Read the model definition and answer for the solid it produces. Units are mm, in the model's axes. A direction names the side the tool comes from. Give positions to 0.01 mm unless a question says otherwise; leave off trailing zeros. Order: outer loops, then holes, each group sorted by start corner. A loop starts at its lowest first (then second) coordinate and runs counter-clockwise, first axis right, second up. Notation, with made-up numbers: M -9.5,-30.75 L 15.5,-30.75 A27 ccw 15.5,-7.75 Z; hole C -32.5,58 d4. An arc over 180 degrees is marked long. Write item = value, one per line. Start each with the question number.
from build123d import *

# Parameters (mm, degrees)
SKETCH_1_W          = 132
SKETCH_1_H          = 40.05
SKETCH_1_R          = 1.6
EXTRUDE_1_DEPTH     = 3
FILLET_1_R          = 5
FILLET_2_R          = 5
SKETCH_4_R          = 1.1
SKETCH_4_W          = 12
SKETCH_4_H          = 19
SKETCH_4_W_2        = 11.2
SKETCH_4_H_2        = 3
CUT_EXTRUDE_1_DEPTH = 10
SKETCH_5_R          = 1.6
SKETCH_5_W          = 5
SKETCH_5_H          = 10
CUT_EXTRUDE_2_DEPTH = 10
FILLET_3_R          = 2


with BuildPart() as part:
    # 草图1 → 凸台-拉伸1 (new body)
    with BuildSketch(Plane(origin=(0, 0, 0), x_dir=(1, 0, 0), z_dir=(0, 1, 0))):
        with Locations((-40.850806452, 4.522983871)):
            Rectangle(SKETCH_1_W, SKETCH_1_H)
        with Locations(Location((18.649193548, 19.647983871, 0), (0, 0, 270))):
            Circle(SKETCH_1_R, mode=Mode.SUBTRACT)
        with Locations(Location((18.649193548, -10.152016129, 0), (0, 0, 270))):
            Circle(SKETCH_1_R, mode=Mode.SUBTRACT)
        with Locations(Location((-5.250806452, 19.647983871, 0), (0, 0, 270))):
            Circle(SKETCH_1_R, mode=Mode.SUBTRACT)
        with Locations(Location((-5.250806452, -10.152016129, 0), (0, 0, 270))):
            Circle(SKETCH_1_R, mode=Mode.SUBTRACT)
        with Locations(Location((-100.350806452, -10.152016129, 0), (0, 0, 90))):
            Circle(SKETCH_1_R, mode=Mode.SUBTRACT)
        with Locations(Location((-76.450806452, -10.152016129, 0), (0, 0, 90))):
            Circle(SKETCH_1_R, mode=Mode.SUBTRACT)
        with Locations(Location((-100.350806452, 19.647983871, 0), (0, 0, 90))):
            Circle(SKETCH_1_R, mode=Mode.SUBTRACT)
        with Locations(Location((-76.450806452, 19.647983871, 0), (0, 0, 90))):
            Circle(SKETCH_1_R, mode=Mode.SUBTRACT)
    extrude(amount=EXTRUDE_1_DEPTH)

    # 圆角1
    fillet_1_edges = [part.edges().sort_by_distance(p)[0] for p in [
        (25.149193548, 1.5, -24.547983871),
    ]]
    fillet(fillet_1_edges, radius=FILLET_1_R)

    # 圆角2
    fillet_2_edges = [part.edges().sort_by_distance(p)[0] for p in [
        (25.149193548, 1.5, 15.502016129),
        (-106.850806452, 1.5, 15.502016129),
        (-106.850806452, 1.5, -24.547983871),
    ]]
    fillet(fillet_2_edges, radius=FILLET_2_R)

    # 草图4 → 切除-拉伸1 (cut)
    with BuildSketch(Plane(origin=(0, 3, 0), x_dir=(1, 0, 0), z_dir=(0, 1, 0))):
        with Locations(Location((4.70662119, 15.172983871, 0), (0, 0, 270))):
            Circle(SKETCH_4_R)
        with Locations(Location((4.799193548, -6.297016129, 0), (0, 0, 270))):
            Circle(SKETCH_4_R)
        with Locations(Location((-15.810806452, 15.092983871, 0), (0, 0, 270))):
            Circle(SKETCH_4_R)
        with Locations(Location((-15.900806452, -6.317016129, 0), (0, 0, 270))):
            Circle(SKETCH_4_R)
        with Locations((16.149193548, 4.522983871)):
            Rectangle(SKETCH_4_W, SKETCH_4_H)
        with Locations((-5.550806452, 16.092983871)):
            Rectangle(SKETCH_4_W_2, SKETCH_4_H_2)
    extrude(amount=-CUT_EXTRUDE_1_DEPTH, mode=Mode.SUBTRACT)

    # 草图5 → 切除-拉伸2 (cut)
    with BuildSketch(Plane(origin=(0, 3, 0), x_dir=(1, 0, 0), z_dir=(0, 1, 0))):
        with Locations(Location((-64.850806452, 15.547983871, 0), (0, 0, 270))):
            Circle(SKETCH_5_R)
        with Locations(Location((-64.850806452, -6.952016129, 0), (0, 0, 270))):
            Circle(SKETCH_5_R)
        with Locations((-27.100806452, 4.522983871)):
            Rectangle(SKETCH_5_W, SKETCH_5_H)
    extrude(amount=-CUT_EXTRUDE_2_DEPTH, mode=Mode.SUBTRACT)

    # 圆角3
    fillet_3_edges = [part.edges().sort_by_distance(p)[0] for p in [
        (-24.600806452, 1.5, 0.477016129),
        (-29.600806452, 1.5, 0.477016129),
        (-29.600806452, 1.5, -9.522983871),
        (-24.600806452, 1.5, -9.522983871),
    ]]
    fillet(fillet_3_edges, radius=FILLET_3_R)


solid = part.part
1) This flat-tipped pin is pushed along its axis until it touches: P1, Ø1.8, axis at x = -15.81, z = -15.09, coming from the -Y side. Where does it stop, or does it pass through?
2) For faces 4 (the face through (23.72, 1.52, 14)), 5 (the face through (22.149, 2, -4)), determine the directions among +Z, -Z, +X, -X, +Y, -Y from which every point of the face is accessible in a straight line to the end or side of a thin tool.
3) Find section A-A on z = 2. Determine the outline of the cut face in (x, y).
4) For a pull along X with two mould halves and no side action, classify faces 1 (the face through (-42, 1, -24.548)), 2 (the face through (-6, 2, -14.593)), 3 (the face through (25.149, 1, -4)) as pulls with the +X half, pulls with the -X half, needs draft (parallel to the pull), parting line crosses it, or undercut.
5) Find section B-B on y = 2.05. Count the separate pieces of the cut face and the enclosed holes in it, plus the area to 3 significant figures.
6) Find the intervals of material crossed by probe 1 along X at (y, z) = (0.85, -7); probe 2 along Z at (x, y) = (-26.5, 0.7); probe 3 along Z at (x, y) = (-9.5, 1.6), in increasing order. Write a range as [from, to].
Numbers:
q1.P1 = through
q2.face_4 = +Z, +X, +Y, -Y
q2.face_5 = +Y, -Y
q3.outline = M -106.85,0 L 10.15,0 L 10.15,3 L -106.85,3 Z; M 22.15,0 L 25.15,0 L 25.15,3 L 22.15,3 Z
q4.face_1 = needs draft
q4.face_2 = undercut
q4.face_3 = pulls with the +X half
q5.separate_pieces = 1
q5.enclosed_holes = 17
q5.area = 4,860 mm2
q6.probe_1 = [-106.85, -29.6], [-24.6, 10.15], [22.15, 25.15]
q6.probe_2 = [-24.55, -9.52], [0.47, 15.5]
q6.probe_3 = [-24.55, -17.59], [-14.59, 15.5]
